Can you work these out from the model? Positions are in its coordinate system, mm. Face numbers are marked on the shaded views. Give positions to 0.01 mm unless a question says otherwise; leave off trailing zeros. Loops run counter-clockwise (first coordinate to the right, second up) from the corner with the lowest first, then second, coordinate; pieces in that order, holes last. Notation, with made-up numbers: (-16.5, 65) - (-8.5, 65) arc R22 ccw to (-8.5, 87) - close; hole circle Ø10 at (-25.5, 87). An arc over 180 degrees is marked (long way). Answer as a JSON object with one key per item and string values. Group by question number.
Item 1: Suppose I cut it at B-B on z = 3. Write out the boundary of the cut face in (x, y).
Item 2: Suppose I cut it at D-D on y = 22. Write out the boundary of the cut face in (x, z), and give its area (3 significant figures).
Item 3: Suppose I cut it at C-C on x = -8. Write out the boundary of the cut face in (y, z).
Item 4: Please list where these lines run through material, in increasing order: L1, parallel to Z at x = -18.5, y = 11.5; L2, parallel to X at y = -45, z = 14.5; L3, parallel to Z at x = -13.5, y = -26.
Item 5: Will these pins go through, and if not, where does the flat tip stop? pin 1 (2 mm diameter, centred on x = -6, y = -13.5, fed in from -Z); pin 2 (6 mm diameter, centred on x = -7.5, y = -39, fed in from -Z); pin 3 (5 mm diameter, centred on x = -21, y = -20.5, fed in from -Z).
Item 6: Suppose I cut it at A-A on x = -27. Write out the boundary of the cut face in (y, z), and give its area (3 significant figures).
Item 7: Thinking about a two-plate mould opening in Y: for the marked faces 1, 2 and 3, which applies, pulls with the +Y half, pulls with the -Y half, needs draft (parallel to the pull), parting line crosses it, or undercut?
from build123d import *

# Parameters (mm, degrees)
F0_R     = 15
F1_DEPTH = 50
F2_R     = 15
F3_DEPTH = 50


with BuildPart() as f1:
    # F0 (on Front) → F1 (new body)
    with BuildSketch(Plane.XZ):
        with Locations((-14.979829, 14.988333)):
            Circle(F0_R)
    extrude(amount=F1_DEPTH)

    # F2 (on Top) → F3 (join)
    with BuildSketch(Plane.XY):
        with Locations((-14.900394, 14.927425)):
            Circle(F2_R)
    extrude(amount=F3_DEPTH)


solid = f1.part
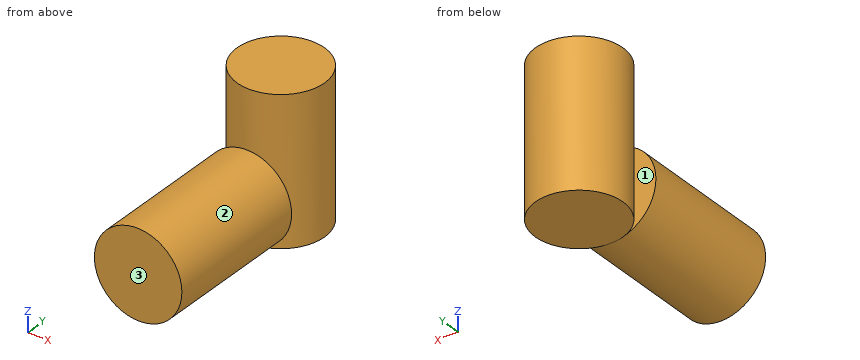
Worked out:
{
 "1": {"outline": "(-24, -50) - (-5.96, -50) - (-5.96, 0) - (-13.43, 0) arc R15 ccw (long way) to (-16.37, 0) - (-24, 0) - close"},
 "2": {"outline": "(-28.13, 0) - (-1.67, 0) - (-1.67, 50) - (-28.13, 50) - close", "area": "1,320 mm2"},
 "3": {"outline": "(-50, 1.71) - (0, 1.71) - (0, 28.27) - (-50, 28.27) - close; (1.61, 0) - (28.25, 0) - (28.25, 50) - (1.61, 50) - close"},
 "4": {"L1": "z = 0 to 50", "L2": "x = -29.97 to 0.01", "L3": "z = 0.06 to 29.92"},
 "5": {"pin 1": "stops at z = 2.29", "pin 2": "stops at z = 0.67", "pin 3": "stops at z = 0.41"},
 "6": {"outline": "(-50, 6.02) - (0, 6.02) - (0, 23.96) - (-50, 23.96) - close; (6.06, 0) - (23.79, 0) - (23.79, 50) - (6.06, 50) - close", "area": "1,780 mm2"},
 "7": {"face 1": "undercut", "face 2": "needs draft", "face 3": "pulls with the -Y half"}
}
